Build history of the part. All positions in model axes, mm. A direction names the side the tool comes from. Coordinates: 2 decimals unless noted, no trailing zeros. Loops run counter-clockwise (first coordinate to the right, second up) from the corner with the lowest first, then second, coordinate; pieces in that order, holes last.
(1) Slice it at A-A (z = 34.65). Give the cut face in (x, y).
(2) Two-plate mould, pull along Z, no slides. Class faces 3 (the face through (2.6, 0, 20)), 4 (the face through (1.804, 19.266, 1.711)), 5 (the face through (1.48, 2.88, 33.48)), 6 (the face through (10, 19, 3)): pulls with the +Z half, pulls with the -Z half, needs draft (parallel to the pull), parting line crosses it, or undercut.
(3) Wall check: L1, parallel to Z at x = 0.7, y = 6.65; L2, parallel to Z at x = 9, y = 19; L3, parallel to Y at x = 10, z = 1.15. Give the ranges that are in metal, low to high.
(4) Flat gauge pins, fed straight in: P1, Ø6, axis at x = 5.5, y = 19, coming from the -Z side; P2, Ø8, axis at x = 10, y = 4, coming from the +Z side; P3, Ø4.5, axis at y = 6.65, z = 47.5, coming from the +X side; P4, Ø1.5, axis at y = 3.25, z = 34.65, coming from the +X side. Where does each tip first touch, or does it go through?
(5) Slice it at B-B (y = 19.5). Give the cut face in (x, z), and give its area (3 significant figures).
(6) Slice it at C-C (y = 29). Give the cut face in (x, z), and give its area (3 significant figures).
(7) Tool access for faces 1 (the face through (2.5, 38, 20.3)), 2 (the face through (3, 19, 19)): list every direction of +Z, -Z, +X, -X, +Y, -Y with a clear straight run to the whole face (end or side of a thin tool).
(8) Slice it at D-D (z = 24). Give the cut face in (x, y), and give its area (3 significant figures).
Autodesk Inventor part; units mm, degrees
ref_plane "YZ Plane" through (0, 0, 0) normal (1, 0, 0) x (0, 1, 0)
ref_plane "XZ Plane" through (0, 0, 0) normal (0, 1, 0) x (-1, 0, 0)
ref_plane "XY Plane" through (0, 0, 0) normal (0, 0, 1) x (1, 0, 0)
sketch "Szkic1" plane through (0, 0, 0) normal (1, 0, 0) x (0, 1, 0)
  line L0 (0, 0) -> (38, 0)
  line L1 (38, 0) -> (38, 52.5)
  line L2 (38, 52.5) -> (0, 52.5)
  line L3 (0, 52.5) -> (0, 0)
  circle A0 centre (19.5, 34.65) radius 12
  circle A1 centre (6.65, 47.5) radius 1.65
  circle A2 centre (32.35, 47.5) radius 1.65
  circle A3 centre (6.65, 21.8) radius 1.65
  circle A4 centre (32.35, 21.8) radius 1.65
  dimension "d0" = 38
  dimension "d1" = 52.5
  dimension "d2" = 24
  dimension "d3" = 17.85
  dimension "d5" = 3.3
  dimension "d6" = 3.3
  dimension "d7" = 3.3
  dimension "d8" = 3.3
  dimension "d9" = 25.7
  dimension "d10" = 25.7
  dimension "d11" = 25.7
  dimension "d12" = 25.7
  dimension "d13" = 5
  dimension "d14" = 5
  dimension "d15" = 12.85
  dimension "d16" = 12.85
  dimension "d38" = 18.5
extrude "Płyta1" add sketch "Szkic1" along normal blind 3
sketch "Szkic2" plane through (0, 38, 3) normal (0, 0, -1) x (-1, 0, 0)
  line L0 (0, -38) -> (0, 0)
  line L1 (0, 0) -> (-15, 0)
  line L2 (-15, 0) -> (-15, -38)
  line L3 (-15, -38) -> (0, -38)
edge flange "Kołnierz1" height 15 angle 90 thickness 3 bend radius 3 thickness toward (0, 0, -1) relief tear relief width 3 relief depth 1.5 edges at (3, 19, 0) wall of the first edge with corners at (0, 0, 3) (0, 38, 3) (15, 38, 3) (15, 0, 3)
bend "Zagięcie1"
corner "Narożnik1"
sketch "Szkic3" plane through (15, 0, 3) normal (0, 0, 1) x (1, 0, 0)
  circle A0 centre (-5, 8) radius 3
  circle A1 centre (-5, 30) radius 3
  line L0 (-9, 38) -> (0, 38)
  line L1 (-9, 0) -> (0, 0)
  line L2 (0, 0) -> (0, 38)
  point P0 (-15, 0)
  dimension "d30" = 6
  dimension "d31" = 6
  dimension "d32" = 8
  dimension "d33" = 8
  dimension "d34" = 5
  dimension "d35" = 5
extrude "Wytnij1" cut sketch "Szkic3" against normal blind 3
chamfer "Fazowanie narożnika1" distance 6 angle 45 1 edges at (15, 0, 1.5)
sketch "Szkic4" plane through (3, 0, 0) normal (1, 0, 0) x (0, 0, -1)
  point P0 (-34.65, 3.2537)
hole "Otwór1" at (3, 3.2537, 34.65) direction (-1, 0, 0) diameter 2.459 depth 3.7451 tip angle 120
equation "\"d36\" = Grubość"
equation "\"d19\" = Grubość"
equation "\"d20\" = SzerokośćGięciaPodcięcia"
equation "\"d21\" = GłębokośćGięciaPodcięcia"
equation "\"d22\" = MinimalnaPozostałość"
equation "\"d23\" = PromieńPrzejścia"
equation "\"d26\" = PromieńGięcia"
equation "\"d27\" = RozmiarPodcięciaNarożnika"
equation "\"d28\" = Wielk_odstępu"
equation "\"d29\" = Rozmiar_promienia_Jacobiego"
equation "\"PromieńGięcia\" = Grubość"
equation "\"SzerokośćGięciaPodcięcia\" = Grubość"
equation "\"GłębokośćGięciaPodcięcia\" = 0.5 * Grubość"
equation "\"RozmiarPodcięciaNarożnika\" = 4 * Grubość"
equation "\"MinimalnaPozostałość\" = 2 * Grubość"
equation "\"PromieńPrzejścia\" = PromieńGięcia"
equation "\"Rozmiar_promienia_Jacobiego\" = PromieńGięcia"
equation "\"Wielk_odstępu\" = Grubość"
properties part number "RR-PCSS-MSK" material "Stal nierdzewna"
Response values:
1. outline: (0, 0) - (3, 0) - (3, 2.02) - (0, 2.02) - close; (0, 4.48) - (3, 4.48) - (3, 7.5) - (0, 7.5) - close; (0, 31.5) - (3, 31.5) - (3, 38) - (0, 38) - close
2. face 3: needs draft
2. face 4: pulls with the -Z half
2. face 5: undercut
2. face 6: pulls with the +Z half
3. L1: z = 3.19 to 20.15, 23.45 to 45.85, 49.15 to 52.5
3. L2: z = 0 to 3
3. L3: y = 1 to 5, 11 to 27, 33 to 38
4. P1: stops at z = 0
4. P2: stops at z = 3
4. P3: stops at x = 3
4. P4: passes through
5. outline: (0, 6) arc R6 ccw to (6, 0) - (15, 0) - (15, 3) - (6, 3) arc R3 cw to (3, 6) - (3, 22.65) - (0, 22.65) - close; (0, 46.65) - (3, 46.65) - (3, 52.5) - (0, 52.5) - close
5. area: 116 mm2
6. outline: (0, 6) arc R6 ccw to (6, 0) - (7.17, 0) - (7.17, 3) - (6, 3) arc R3 cw to (3, 6) - (3, 27.32) - (0, 27.32) - close; (0, 41.98) - (3, 41.98) - (3, 52.5) - (0, 52.5) - close; (12.83, 0) - (15, 0) - (15, 3) - (12.83, 3) - close
6. area: 127 mm2
7. face 1: +Z, -Z, +X, -X, +Y
7. face 2: +Z, +X, +Y, -Y
8. outline: (0, 0) - (3, 0) - (3, 13.97) - (0, 13.97) - close; (0, 25.03) - (3, 25.03) - (3, 38) - (0, 38) - close
8. area: 80.8 mm2
